Design review of the part shown in the three views and the two pictorial views. Dimensions are in mm from the part's minimum x, y and z. Round coordinates to 2 decimals unless told otherwise and drop trailing zeros. Order: outer loops, then holes, each group sorted by start corner. A loop starts at its lowest first (then second) coordinate and runs counter-clockwise, first axis right, second up.
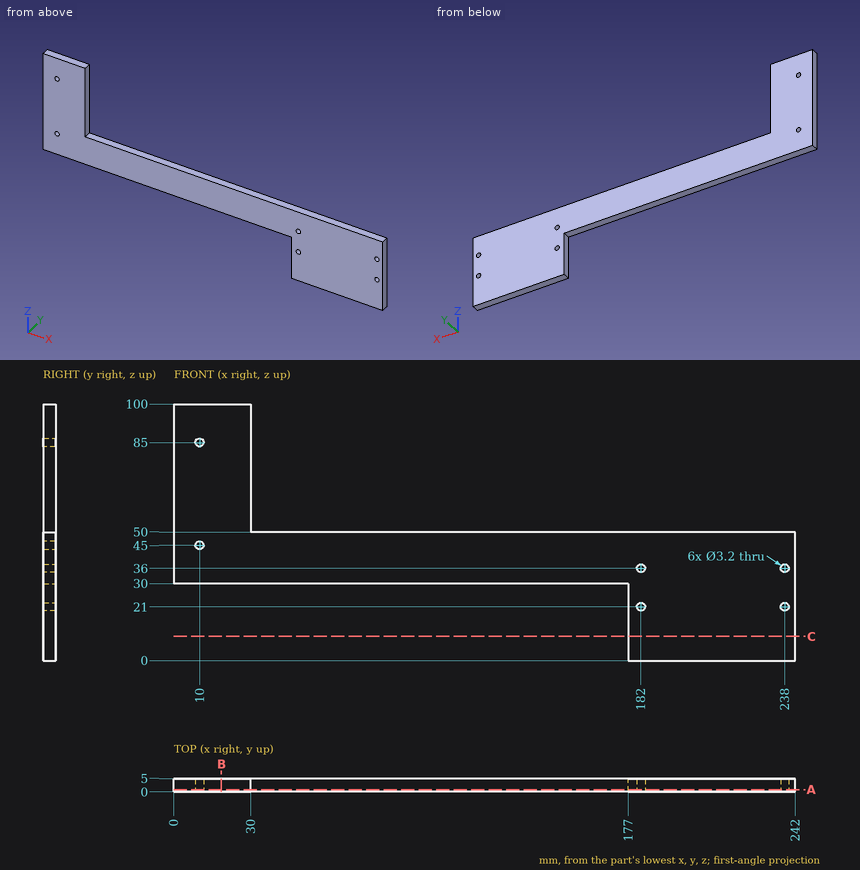
(1) To check wall thickness, follow probe 1 along X at (y, z) = (2.2, 36); probe 2 along X at (y, z) = (1.3, 21); probe 3 along Z at (x, y) = (182, 2.75). State the ranges of each line that lie inside material, in increasing order.
Data:
probe 1: x = 0 to 180.4, 183.6 to 236.4, 239.6 to 242
probe 2: x = 177 to 180.4, 183.6 to 236.4, 239.6 to 242
probe 3: z = 0 to 19.4, 22.6 to 34.4, 37.6 to 50
(2) Consider section C-C (z = 9.5). Write out the cut boundary in (x, y).
Data:
outline: (177, 0) - (242, 0) - (242, 5) - (177, 5) - close
(3) Insertion check: pin 1 (2.5 mm diameter, centred on x = 91.5, y = 1.5, fed in from -Z); pin 2 (3.5 mm diameter, centred on x = 182, z = 21, fed in from -Y); pin 3 (2.5 mm diameter, centred on y = 2.5, z = 63.5, fed in from +X); pin 4 (1.5 mm diameter, centred on x = 132.5, y = 3, fed in from +Z). Each pin has a flat end and moves straight along its axis. Give the tip position at first contact, or say it passes through.
Data:
pin 1: stops at z = 30
pin 2: stops at y = 0
pin 3: stops at x = 30
pin 4: stops at z = 50
(4) Consider section B-B (x = 18.5). Write out the cut boundary in (y, z), and give its area (3 significant figures).
Data:
outline: (0, 30) - (5, 30) - (5, 100) - (0, 100) - close
area: 350 mm2
(5) Consider section A-A (y = 0.75). Write out the cut boundary in (x, z).
Data:
outline: (0, 30) - (177, 30) - (177, 0) - (242, 0) - (242, 50) - (30, 50) - (30, 100) - (0, 100) - close; hole circle Ø3.2 at (10, 45); hole circle Ø3.2 at (10, 85); hole circle Ø3.2 at (182, 21); hole circle Ø3.2 at (182, 36); hole circle Ø3.2 at (238, 21); hole circle Ø3.2 at (238, 36)
